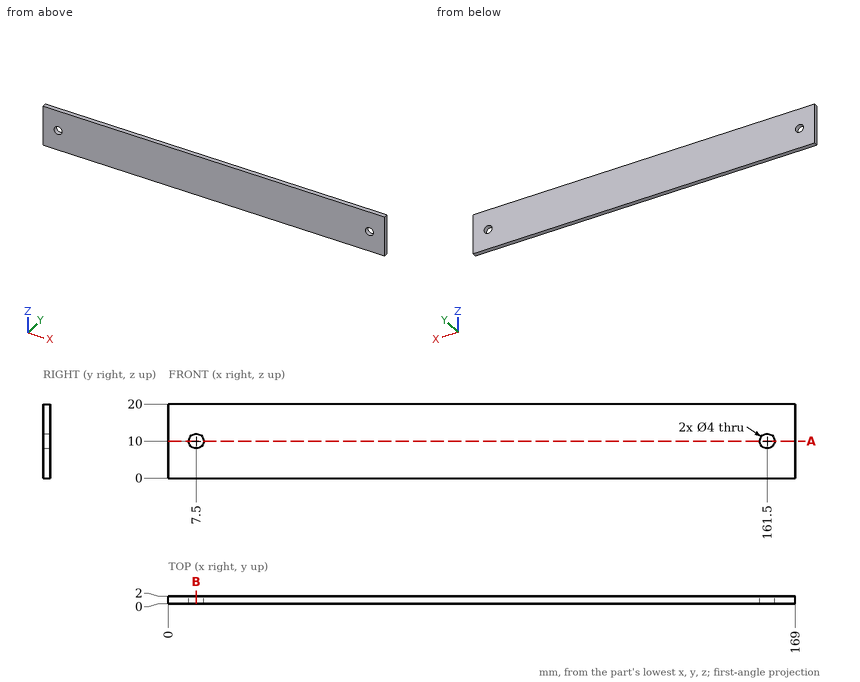
Verification items for this drawing (mm, ordinates from the low corner). Coordinates: 2 decimals unless noted, no trailing zeros. Loops run counter-clockwise (first coordinate to the right, second up) from the corner with the lowest first, then second, coordinate; pieces in that order, holes last.
Item 1: Thickness scan on line 1 (X direction, y = 1.5, z = 10); line 2 (Z direction, x = 7.5, y = 1.25); line 3 (X direction, y = 0.95, z = 8.5). Record the ranges inside material, lowest first.
Item 2: Go/stop test with a flat-tipped pin: pin 1 Ø2.5 at (x, z) = (7.5, 10) entering from +Y. Record where the tip stops, or that it passes through.
Item 3: Sectioned sample at B-B, the plane x = 7.5. Record the boundary of the cut face in (y, z), then the cut area to 3 significant figures.
Item 4: Sectioned sample at A-A, the plane z = 10. Record the boundary of the cut face in (x, y).
Check result:
1. line 1: x = 0 to 5.5, 9.5 to 159.5, 163.5 to 169
1. line 2: z = 0 to 8, 12 to 20
1. line 3: x = 0 to 6.18, 8.82 to 160.18, 162.82 to 169
2. pin 1: passes through
3. outline: (0, 0) - (2, 0) - (2, 8) - (0, 8) - close; (0, 12) - (2, 12) - (2, 20) - (0, 20) - close
3. area: 32.0 mm2
4. outline: (0, 0) - (5.5, 0) - (5.5, 2) - (0, 2) - close; (9.5, 0) - (159.5, 0) - (159.5, 2) - (9.5, 2) - close; (163.5, 0) - (169, 0) - (169, 2) - (163.5, 2) - close
